The model under review builds one solid part; all positions refer to its coordinate system, in mm. A direction names the side the tool comes from. Coordinates: 2 decimals unless noted, no trailing zeros. Write each loop counter-clockwise with the first axis right and the second up, starting at its lowest first coordinate (ties: lowest second). Pieces come first, ordered by that corner, then holes.
```python
from build123d import *

# Parameters (mm, degrees)
SKETCH9_W           = 5.5
SKETCH9_H           = 12.5
BOSS_EXTRUDE1_DEPTH = 4
SKETCH11_W          = 6.5
SKETCH11_H          = 12.5
SKETCH11_W_2        = 12
SKETCH11_H_2        = 18.5
BOSS_EXTRUDE2_DEPTH = 2
BOSS_EXTRUDE3_DEPTH = 2
BOSS_EXTRUDE4_DEPTH = 35


with BuildPart() as part:
    # Sketch9 → Boss-Extrude1 (new body)
    with BuildSketch(Plane(origin=(0, 3, 0), x_dir=(1, 0, 0), z_dir=(0, 1, 0))):
        Polygon((0, -3), (0, 0), (-6.5, 0), (-12, 0), (-12, -3), align=None)
        with Locations((-9.25, 6.25)):
            Rectangle(SKETCH9_W, SKETCH9_H)
        Polygon((-6.5, 12.5), (0, 12.5), (0, 15.5), (-12, 15.5), (-12, 12.5), align=None)
        Polygon((130, 15.5), (130, 12.5), (136.5, 12.5), (142, 12.5), (142, 15.5), align=None)
        with Locations((139.25, 6.25)):
            Rectangle(SKETCH9_W, SKETCH9_H)
        Polygon((136.5, 0), (130, 0), (130, -3), (142, -3), (142, 0), align=None)
        Polygon((136.5, 95.5), (130, 95.5), (130, 92.5), (142, 92.5), (142, 95.5), align=None)
        with Locations((139.25, 101.75)):
            Rectangle(SKETCH9_W, SKETCH9_H)
        Polygon((130, 111), (130, 108), (136.5, 108), (142, 108), (142, 111), align=None)
        Polygon((0, 92.5), (0, 95.5), (-6.5, 95.5), (-12, 95.5), (-12, 92.5), align=None)
        with Locations((-9.25, 101.75)):
            Rectangle(SKETCH9_W, SKETCH9_H)
        Polygon((-6.5, 108), (0, 108), (0, 111), (-12, 111), (-12, 108), align=None)
    extrude(amount=BOSS_EXTRUDE1_DEPTH)

    # Sketch11 → Boss-Extrude2 (add)
    with BuildSketch(Plane.XZ.offset(-3)):
        Polygon((130, 0), (0, 0), (0, -12.5), (0, -15.5), (0, -92.5), (0, -108), (130, -108), (130, -92.5), (130, -15.5), align=None)
        with Locations((-3.25, -6.25)):
            Rectangle(SKETCH11_W, SKETCH11_H)
        Polygon((-6.5, -12.5), (-6.5, 0), (0, 0), (0, 3), (-12, 3), (-12, -15.5), (0, -15.5), (0, -12.5), align=None)
        with Locations((136, -6.25)):
            Rectangle(SKETCH11_W_2, SKETCH11_H_2)
        with Locations((136, -101.75)):
            Rectangle(SKETCH11_W_2, SKETCH11_H_2)
        with Locations((-6, -101.75)):
            Rectangle(SKETCH11_W_2, SKETCH11_H_2)
    extrude(amount=BOSS_EXTRUDE2_DEPTH)

    # Sketch12 → Boss-Extrude3 (add)
    with BuildSketch(Plane.XZ.offset(-1)):
        Polygon((12.5, -119.5), (12.5, -108), (0, -108), (0, -111), (0, -119.5), align=None)
        Polygon((0, 0), (12.5, 0), (12.5, 12.5), (0, 12.5), (0, 3), align=None)
        Polygon((117.5, 0), (130, 0), (130, 3), (130, 12.5), (117.5, 12.5), align=None)
        Polygon((130, -111), (130, -108), (117.5, -108), (117.5, -119.5), (130, -119.5), align=None)
    extrude(amount=-BOSS_EXTRUDE3_DEPTH)

    # Sketch13 → Boss-Extrude4 (add)
    with BuildSketch(Plane(origin=(0, 1, 0), x_dir=(-1, 0, 0), z_dir=(0, -1, 0))):
        Polygon((-12.5, -12.5), (0, -12.5), (0, -3), (0, 0), (-12.5, 0), align=None)
        Polygon((0, 0), (0, -3), (12, -3), (12, 15.5), (0, 15.5), align=None)
        Polygon((-117.5, -12.5), (-117.5, 0), (-130, 0), (-130, -3), (-130, -12.5), align=None)
        Polygon((-130, -3), (-130, 0), (-130, 15.5), (-142, 15.5), (-142, -3), align=None)
        Polygon((-142, 92.5), (-130, 92.5), (-130, 108), (-130, 111), (-142, 111), align=None)
        Polygon((-130, 111), (-130, 108), (-117.5, 108), (-117.5, 119.5), (-130, 119.5), align=None)
        Polygon((-12.5, 108), (0, 108), (0, 111), (0, 119.5), (-12.5, 119.5), align=None)
        Polygon((0, 108), (0, 92.5), (12, 92.5), (12, 111), (0, 111), align=None)
    extrude(amount=BOSS_EXTRUDE4_DEPTH)


solid = part.part
```
Item 1: For pin 1 (3.5 mm diameter, centred on x = 133.5, y = -18.5, fed in from -Z); pin 2 (8 mm diameter, centred on x = 29.5, z = -105.5, fed in from +Y); pin 3 (1 mm diameter, centred on x = 76.5, z = -19.5, fed in from -Y); pin 4 (2 mm diameter, centred on x = 114, y = -1, fed in from +Z), all flat-tipped, find the tip position at first contact; note any pin that passes through.
Solved:
pin 1: stops at z = -111
pin 2: stops at y = 3
pin 3: stops at y = 1
pin 4: passes through
Item 2: Mouldability with a two-part tool opening along X and no side actions: class faces 6 (the face through (133, 5, 0)), 7 (the face through (0, -15, 8)), 8 (the face through (133, -34, -2)), 9 (the face through (142, -13, -102)) as pulls with the +X half, pulls with the -X half, needs draft (parallel to the pull), parting line crosses it, or undercut.
Solved:
face 6: undercut
face 7: pulls with the -X half
face 8: needs draft
face 9: pulls with the +X half
Item 3: Take a section at C-C, the plane x = 24. Write out the cut boundary in (y, z), plus the area to 3 significant figures.
Solved:
outline: (1, -108) - (3, -108) - (3, 0) - (1, 0) - close
area: 216 mm2
Item 4: Take a section at D-D, the plane z = -37.5. Write out the cut boundary in (x, y).
Solved:
outline: (0, 1) - (130, 1) - (130, 3) - (0, 3) - close
Item 5: Machinability: for faces 1 (the face through (136.5, 5, -6)), 2 (the face through (-6, -13, -111)), 3 (the face through (137, 7, -102)), 4 (the face through (124, -16, -108)), 5 (the face through (124, -16, -119.5)), which of the approach directions +Z, -Z, +X, -X, +Y, -Y give a long, thin tool a straight path to every point of the face, cutting with its end or side? Answer none if there is none.
Solved:
face 1: +Y
face 2: -Z, -X, +Y, -Y
face 3: +Z, -Z, +X, -X, +Y
face 4: -Y
face 5: -Z, +X, -X, +Y, -Y
Item 6: Take a section at B-B, the plane z = -106. Write out the cut boundary in (x, y).
Solved:
outline: (-12, -34) - (0, -34) - (0, 1) - (130, 1) - (130, -34) - (142, -34) - (142, 7) - (136.5, 7) - (136.5, 3) - (-6.5, 3) - (-6.5, 7) - (-12, 7) - close
Item 7: To check wall thickness, follow line 1 along X through (y, z) = (-22, -2.5); line 2 along Z through (x, y) = (128, -29.5); line 3 along X through (y, z) = (-9.5, -108.5). State the ranges of each line that lie inside material, in increasing order.
Solved:
line 1: x = -12 to 0, 130 to 142
line 2: z = -119.5 to -108, 0 to 12.5
line 3: x = -12 to 12.5, 117.5 to 142
Item 8: Take a section at A-A, the plane y = -8. Count the separate pieces of the cut face and the enclosed holes in it, plus the area to 3 significant figures.
Solved:
separate pieces: 4
enclosed holes: 0
area: 1,490 mm2
